```python
from build123d import *

# Parameters (mm, degrees)
SKETCH1_R           = 17.5
SKETCH1_R_2         = 1.5
SKETCH1_R_3         = 7.5
BOSS_EXTRUDE1_DEPTH = 3
SKETCH3_R           = 15
SKETCH3_R_2         = 12
BOSS_EXTRUDE2_DEPTH = 1.5
CHAMFER1_SIZE       = 0.5


with BuildPart() as part:
    # Sketch1 → Boss-Extrude1 (new body, symmetric)
    with BuildSketch(Plane(origin=(0, 0, 0), x_dir=(1, 0, 0), z_dir=(0, 1, 0))):
        Circle(SKETCH1_R)
        with Locations((13.5, 0)):
            Circle(SKETCH1_R_2, mode=Mode.SUBTRACT)
        with Locations((6.75, -11.691342951)):
            Circle(SKETCH1_R_2, mode=Mode.SUBTRACT)
        with Locations((-6.75, -11.691342951)):
            Circle(SKETCH1_R_2, mode=Mode.SUBTRACT)
        with Locations((-13.5, 0)):
            Circle(SKETCH1_R_2, mode=Mode.SUBTRACT)
        with Locations((-6.75, 11.691342951)):
            Circle(SKETCH1_R_2, mode=Mode.SUBTRACT)
        with Locations((6.75, 11.691342951)):
            Circle(SKETCH1_R_2, mode=Mode.SUBTRACT)
        Circle(SKETCH1_R_3, mode=Mode.SUBTRACT)
    extrude(amount=BOSS_EXTRUDE1_DEPTH, both=True)

    # Sketch3 → Boss-Extrude2 (add)
    with BuildSketch(Plane.XZ.offset(3)):
        Circle(SKETCH3_R)
        Circle(SKETCH3_R_2, mode=Mode.SUBTRACT)
    extrude(amount=-BOSS_EXTRUDE2_DEPTH)

    # Chamfer1
    chamfer1_edges = [part.edges().sort_by_distance(p)[0] for p in [
        (-7.5, -3, 0),
        (-7.5, 3, 0),
    ]]
    chamfer(chamfer1_edges, length=CHAMFER1_SIZE)


solid = part.part
```
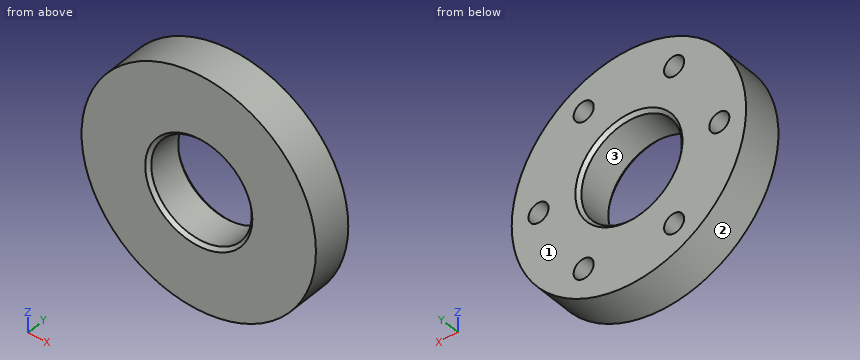
CAD build for the part. Positions are in the model's coordinates, mm. Face numbers are marked on the shaded views. Round coordinates to 2 decimals unless told otherwise and drop trailing zeros. Order: outer loops, then holes, each group sorted by start corner. A loop starts at its lowest first (then second) coordinate and runs counter-clockwise, first axis right, second up. Notation, with made-up numbers: (31, -2.5) - (66, -2.5) arc R12 cw to (66, 9.5) - close; hole circle Ø6 at (40.5, 1). An arc over 180 degrees is marked (long way). Answer in a Markdown table with one row per item. Add a question column.
(1) Band-saw the part on A-A on x = 0. List the corners of the cut face in (y, z).
(2) Probe L1, parallel to X at y = -0.5, z = 0; L2, parallel to X at y = -0.5, z = -12; L3, parallel to Z at x = -6.75, y = 1.55. List the from-to ranges inside material, lowest first. Write a range as [from, to].
(3) Band-saw the part on B-B on z = 0. List the corners of the cut face in (x, y).
(4) Drop flat-ended pins along their axis: pin 1 Ø3 at (x, y) = (-4, 0.5) entering from -Z; pin 2 Ø0.9 at (x, z) = (7, -11.5) entering from +Y; pin 3 Ø1 at (x, y) = (-7, -0.5) entering from +Z. Give the stop position or say it passes through.
(5) Band-saw the part on D-D on x = -13.5. List the corners of the cut face in (y, z), and give its area (3 significant figures).
(6) Mould opens along X. For the marked faces 1, 2 and 3 say: +X half, -X half, draft (parallel to the pull), parting line (faces both ways), or undercut.
(7) Band-saw the part on C-C on y = -0.8. List the corners of the cut face in (x, z), and give its area (3 significant figures).
Data:
| question | item | result |
|---|---|---|
| 1 | outline | (-3, -17.5) - (3, -17.5) - (3, -8) - (2.5, -7.5) - (-2.5, -7.5) - (-3, -8) - close; (-3, 8) - (-2.5, 7.5) - (2.5, 7.5) - (3, 8) - (3, 17.5) - (-3, 17.5) - close |
| 2 | L1 | x = [-17.5, -15], [-12, -7.5], [7.5, 12], [15, 17.5] |
| 2 | L2 | x = [-12.74, -8.22], [-5.28, 5.28], [8.22, 12.74] |
| 2 | L3 | z = [-16.15, -13.19], [-10.19, -3.27], [3.27, 10.19], [13.19, 16.15] |
| 3 | outline | (-17.5, -3) - (-8, -3) - (-7.5, -2.5) - (-7.5, 2.5) - (-8, 3) - (-12, 3) - (-12, -1.5) - (-15, -1.5) - (-15, 3) - (-17.5, 3) - close; (7.5, -2.5) - (8, -3) - (17.5, -3) - (17.5, 3) - (15, 3) - (15, -1.5) - (12, -1.5) - (12, 3) - (8, 3) - (7.5, 2.5) - close |
| 4 | pin 1 | stops at z = -17.32 |
| 4 | pin 2 | stops at y = -1.5 |
| 4 | pin 3 | stops at z = 16.25 |
| 5 | outline | (-3, -11.14) - (3, -11.14) - (3, -1.5) - (-1.5, -1.5) - (-1.5, 1.5) - (3, 1.5) - (3, 11.14) - (-3, 11.14) - close |
| 5 | area | 120 mm^2 |
| 6 | face 1 | draft |
| 6 | face 2 | parting line |
| 6 | face 3 | undercut |
| 7 | outline | circle Ø35 at (0, 0); hole circle Ø3 at (-13.5, 0); hole circle Ø3 at (-6.75, -11.69); hole circle Ø3 at (-6.75, 11.69); hole circle Ø15 at (0, 0); hole circle Ø3 at (6.75, -11.69); hole circle Ø3 at (6.75, 11.69); hole circle Ø3 at (13.5, 0) |
| 7 | area | 743 mm^2 |
